```python
from build123d import *

# Parameters (mm, degrees)
SKETCH2_R           = 38.1
BOSS_EXTRUDE2_DEPTH = 25.4
FILLET3_R           = 7.62
FILLET5_R           = 7.62
SKETCH4_R           = 1.7
CUT_EXTRUDE1_DEPTH  = 25.4
CUT_EXTRUDE2_DEPTH  = 4


with BuildPart() as part:
    # Sketch2 → Boss-Extrude2 (new body)
    with BuildSketch(Plane(origin=(0, 0, 0), x_dir=(0, 0, -1), z_dir=(1, 0, 0))):
        Circle(SKETCH2_R)
    extrude(amount=BOSS_EXTRUDE2_DEPTH)

    # Fillet3
    fillet3_edges = [part.edges().sort_by_distance(p)[0] for p in [
        (25.4, 0, 38.1),
    ]]
    fillet(fillet3_edges, radius=FILLET3_R)

    # Fillet5
    fillet5_edges = [part.edges().sort_by_distance(p)[0] for p in [
        (0, 0, 38.1),
    ]]
    fillet(fillet5_edges, radius=FILLET5_R)

    # Sketch4 → Cut-Extrude1 (cut)
    with BuildSketch(Plane(origin=(25.4, 0, 0), x_dir=(0, 0, -1), z_dir=(1, 0, 0))):
        Circle(SKETCH4_R)
    extrude(amount=-CUT_EXTRUDE1_DEPTH, mode=Mode.SUBTRACT)

    # Sketch5 → Cut-Extrude2 (cut)
    with BuildSketch(Plane(origin=(25.4, 0, 0), x_dir=(0, 0, -1), z_dir=(1, 0, 0))):
        Polygon((-3.387274931, 2.13272866), (-3.540634665, -1.86710181), (-0.153359734, -3.99983047), (3.387274931, -2.13272866), (3.540634665, 1.86710181), (0.153359734, 3.99983047), align=None)
    extrude(amount=-CUT_EXTRUDE2_DEPTH, mode=Mode.SUBTRACT)


solid = part.part
```
Model file for the job. Use its own axes, mm. A direction names the side the tool comes from. Coordinates: 2 decimals unless noted, no trailing zeros. Loops run counter-clockwise (first coordinate to the right, second up) from the corner with the lowest first, then second, coordinate; pieces in that order, holes last. Notation, with made-up numbers: (84, -37.75) - (100, -37.75) arc R22 cw to (100, -28.75) - close; hole circle Ø4 at (-35.75, 63.25). An arc over 180 degrees is marked (long way). Answer as a JSON object with one key per item and string values. Group by question number.
(1) Cut at C-C (x = 19). Give the cut face in (y, z), then the cut area to 3 significant figures.
(2) Cut at A-A (y = 0). Give the cut face in (x, z).
(3) Cut at B-B (x = 15). Give the cut face in (y, z), then the cut area to 3 significant figures.
(4) Flat gauge pins, fed straight in: pin 1 (4 mm diameter, centred on x = 20, z = 20.5, fed in from +Y); pin 2 (1 mm diameter, centred on x = 19.5, y = 14.5, fed in from -Z); pin 3 (1.5 mm diameter, centred on x = 10, y = -22, fed in from -Z); pin 4 (5 mm diameter, centred on y = 22, z = -15, fed in from -X). Where does each tip first touch, or does it go through?
(5) Tool access for faces 4 (the face through (21.4, -2, 0)), 5 (the face through (25.4, -6, 0)): list every direction of +Z, -Z, +X, -X, +Y, -Y with a clear straight run to the whole face (end or side of a thin tool).
(6) Probe line 1 along Y through (x, z) = (17, 0); line 2 along Y through (x, z) = (5.25, 0); line 3 along X through (y, z) = (-31, 7). List the from-to ranges inside material, lowest first.
(7) Two-plate mould, pull along Z, no slides. Class faces 1 (the face through (0, -6, 0)), 2 (the face through (12.629, -23.183, 30.235)), 3 (the face through (10.85, -1.66, 0.37)): released by +Z, released by -Z, zero draft, split by the parting line, or undercut.
Geometry says:
{
 "1": {"outline": "circle Ø76 at (0, 0); hole circle Ø3.4 at (0, 0)", "area": "4,530 mm^2"},
 "2": {"outline": "(0, -30.48) arc R7.62 ccw to (7.62, -38.1) - (17.78, -38.1) arc R7.62 ccw to (25.4, -30.48) - (25.4, -3.47) - (21.4, -3.47) - (21.4, -1.7) - (0, -1.7) - close; (0, 1.7) - (21.4, 1.7) - (21.4, 3.47) - (25.4, 3.47) - (25.4, 30.48) arc R7.62 ccw to (17.78, 38.1) - (7.62, 38.1) arc R7.62 ccw to (0, 30.48) - close"},
 "3": {"outline": "circle Ø76.2 at (0, 0); hole circle Ø3.4 at (0, 0)", "area": "4,550 mm^2"},
 "4": {"pin 1": "stops at y = 33.06", "pin 2": "stops at z = -35.25", "pin 3": "stops at z = -31.62", "pin 4": "stops at x = 0"},
 "5": {"face 4": "+X", "face 5": "+Z, -Z, +X, +Y, -Y"},
 "6": {"line 1": "y = -38.1 to -1.7, 1.7 to 38.1", "line 2": "y = -37.72 to -1.7, 1.7 to 37.72", "line 3": "x = 0.11 to 25.29"},
 "7": {"face 1": "zero draft", "face 2": "split by the parting line", "face 3": "undercut"}
}
